from build123d import *

# Parameters (mm, degrees)
F0_W   = 28.4530296922
F0_H   = 13.0855888128
F0_W_2 = 34.8043181002
F0_H_2 = 13.3176594973
F2_R   = 10


with BuildPart() as f1:
    # F0 (on Front) → F1 (revolve)
    with BuildSketch(Plane.XZ):
        with Locations((-14.2265148461, 65.3495416045)):
            Rectangle(F0_W, F0_H)
        Polygon((0, -58.8067471981), (0, 58.8067471981), (-28.4530296922, 58.8067471981), (-65.5450373888, 58.8067471981), (-65.5450373888, -58.8067471981), (-34.8043181002, -58.8067471981), align=None)
        with Locations((-17.4021590501, -65.4655769467)):
            Rectangle(F0_W_2, F0_H_2)
    revolve(axis=Axis((0, 0, 0), (0, 0, -1)))

    # F2
    f2_edges = [f1.edges().sort_by_distance(p)[0] for p in [
        (65.545037, 0, 58.806747),
        (65.545037, 0, -58.806747),
        (-65.545037, 0, 0),
    ]]
    fillet(f2_edges, radius=F2_R)


solid = f1.part
The listing builds one solid part. Answer for the finished solid, in the listing's coordinates (mm). A direction names the side the tool comes from. Give positions to 0.01 mm unless a question says otherwise; leave off trailing zeros. Order: outer loops, then holes, each group sorted by start corner. A loop starts at its lowest first (then second) coordinate and runs counter-clockwise, first axis right, second up. Notation, with made-up numbers: (9.25, -19.75) - (29.25, -19.75) arc R17 cw to (29.25, -10.75) - close; hole circle Ø10 at (-8.75, 84). An arc over 180 degrees is marked (long way). Answer as CSV lines item,"result".
Q1. A cutting plane is placed at B-B, the plane z = 41. Determine the outline of the cut face in (x, y).
Answer key:
outline,"circle Ø131.09 at (0, 0)"
Q2. Each of these flat-tipped pins is pushed along its axis until it touches: pin 1 Ø5 at (x, z) = (17.5, -7.5) entering from +Y; pin 2 Ø12 at (x, z) = (40.5, -4) entering from -Y; pin 3 Ø10 at (y, z) = (38, 14.5) entering from -X; pin 4 Ø12 at (x, y) = (34, -8) entering from -Z. Where does it stop, or does it pass through?
Answer key:
pin 1,"stops at y = 63.81"
pin 2,"stops at y = -55.73"
pin 3,"stops at x = -56.63"
pin 4,"stops at z = -72.12"
Q3. A cutting plane is placed at A-A, the plane y = 0. Determine the outline of the cut face in (x, z), and give its area (3 significant figures).
Answer key:
outline,"(-65.55, -48.81) arc R10 ccw to (-55.55, -58.81) - (-34.8, -58.81) - (-34.8, -72.12) - (34.8, -72.12) - (34.8, -58.81) - (55.55, -58.81) arc R10 ccw to (65.55, -48.81) - (65.55, 48.81) arc R10 ccw to (55.55, 58.81) - (28.45, 58.81) - (28.45, 71.89) - (-28.45, 71.89) - (-28.45, 58.81) - (-55.55, 58.81) arc R10 ccw to (-65.55, 48.81) - close"
area,"17,000 mm^2"
Q4. Straight lines are drawn through the part: L1, parallel to Z at x = 45.5, y = 7; L2, parallel to X at y = -8, z = -14 (3 decimals); L3, parallel to Y at x = 42.5, z = -9.5. For each, find the intervals that lie inside material, in ascending order.
Answer key:
L1,"z = -58.81 to 58.81"
L2,"x = -65.055 to 65.055"
L3,"y = -49.9 to 49.9"
Q5. Which of the six approach directions +Z, -Z, +X, -X, +Y, -Y give full straight-line access (tool end or side, diameter ignored) to faces 1 (the face through (1, -36, -58.807)), 2 (the face through (-25.5, 13.1, 58.807)), 3 (the face through (0, 0, 71.892))?
Answer key:
face 1,"-Z"
face 2,"+Z"
face 3,"+Z, +X, -X, +Y, -Y"
